from build123d import *

# Parameters (mm, degrees)
ESTRUSIONE_ESTRUSIONE1_DEPTH      = 30
ESTRUSIONE_ESTRUSIONE1_DEPTH_BACK = 6
SCHIZZO1_W                        = 3
SCHIZZO1_H                        = 40
SCHIZZO2_W                        = 3
SCHIZZO2_H                        = 30
ESTRUSIONE_ESTRUSIONE2_DEPTH      = 10


with BuildPart() as part:
    # Schizzo1 → Estrusione-Estrusione1 (new, two sides: drawn at the far end of the back side and taken through both)
    with BuildSketch(Plane.XY.offset(1).offset(-ESTRUSIONE_ESTRUSIONE1_DEPTH_BACK)):
        with Locations((71.042298103, 0)):
            Rectangle(SCHIZZO1_W, SCHIZZO1_H)
    extrude(amount=ESTRUSIONE_ESTRUSIONE1_DEPTH + ESTRUSIONE_ESTRUSIONE1_DEPTH_BACK)

    # Schizzo2 → Estrusione-Estrusione2 (add)
    with BuildSketch(Plane(origin=(0, 20, 0), x_dir=(1, 0, 0), z_dir=(0, 1, 0))):
        with Locations((71.042298103, -16)):
            Rectangle(SCHIZZO2_W, SCHIZZO2_H)
    estrusione_estrusione2 = extrude(amount=ESTRUSIONE_ESTRUSIONE2_DEPTH)

    # Specchia1: Estrusione-Estrusione2 across plane
    add(estrusione_estrusione2.mirror(Plane.ZX))


solid = part.part
Input: part model. Units: mm. Frame: model coordinates. A direction names the side the tool comes from. Round coordinates to 2 decimals unless told otherwise and drop trailing zeros. Order: outer loops, then holes, each group sorted by start corner. A loop starts at its lowest first (then second) coordinate and runs counter-clockwise, first axis right, second up.
1. Material intervals for line 1 (Z direction, x = 70.95, y = 22); line 2 (Y direction, x = 71, z = 0), sorted ascending.
The answers:
line 1: z = 1 to 31
line 2: y = -20 to 20
2. Cut plane B-B, the plane y = 23. Output: boundary loops of the cut face in (x, z), then the cut area to 3 significant figures.
The answers:
outline: (69.54, 1) - (72.54, 1) - (72.54, 31) - (69.54, 31) - close
area: 90.0 mm2
3. Set-up query: faces 1 (the face through (71, 0, -5)), 2 (the face through (71, 20, -2)), 3 (the face through (71, -25, 1)). Return all of +Z, -Z, +X, -X, +Y, -Y with unobstructed straight access to the full face (end or side cutting, diameter ignored); none if empty.
The answers:
face 1: -Z, +X, -X, +Y, -Y
face 2: -Z, +X, -X, +Y
face 3: -Z, +X, -X, -Y
4. Pin query (flat end, axial travel): P1, Ø0.9, axis at x = 71.5, z = -1.5, coming from the -Y side; P2, Ø0.9, axis at x = 71.5, z = -1.5, coming from the +Y side. Return the tip coordinate at first contact, or that it passes through.
The answers:
P1: stops at y = -20
P2: stops at y = 20
5. Cut plane A-A, the plane x = 70.6. Output: boundary loops of the cut face in (y, z), then the cut area to 3 significant figures.
The answers:
outline: (-30, 1) - (-20, 1) - (-20, -5) - (20, -5) - (20, 1) - (30, 1) - (30, 31) - (-30, 31) - close
area: 2,040 mm2
